from build123d import *

# Parameters (mm, degrees)
SKETCH_1_R          = 14
SKETCH_1_R_2        = 8.2
EXTRUDE_1_DEPTH     = 6
EXTRUDE_2_DEPTH     = 16
SKETCH_3_R          = 1.7
CUT_EXTRUDE_1_DEPTH = 34.540015912
SKETCH_4_R          = 1.5
CUT_EXTRUDE_2_DEPTH = 34.540015912
CUT_EXTRUDE_3_DEPTH = 13
CHAMFER_1_SIZE      = 3
CHAMFER_2_SIZE      = 1


with BuildPart() as part:
    # 草圖1 → 填料-伸長1 (new body)
    with BuildSketch(Plane.XY):
        Circle(SKETCH_1_R)
        Circle(SKETCH_1_R_2, mode=Mode.SUBTRACT)
    extrude(amount=EXTRUDE_1_DEPTH)

    # 草圖2 → 填料-伸長2 (add)
    with BuildSketch(Plane.XY):
        with BuildLine():
            Line((20.686533479, -6.169872981), (13.824751653, -2.208221396))
            ThreePointArc((13.824751653, -2.208221396), (12.124355653, -7), (8.824751653, -10.868475434))
            Line((8.824751653, -10.868475434), (15.686533479, -14.830127019))
            Line((15.686533479, -14.830127019), (20.686533479, -6.169872981))
        make_face()
        with BuildLine():
            Line((-5, 21), (5, 21))
            Line((5, 21), (5, 13.076696831))
            ThreePointArc((5, 13.076696831), (0, 14), (-5, 13.076696831))
            Line((-5, 13.076696831), (-5, 21))
        make_face()
        with BuildLine():
            Line((-15.686533479, -14.830127019), (-8.824751653, -10.868475434))
            ThreePointArc((-8.824751653, -10.868475434), (-12.124355653, -7), (-13.824751653, -2.208221396))
            Line((-13.824751653, -2.208221396), (-20.686533479, -6.169872981))
            Line((-20.686533479, -6.169872981), (-15.686533479, -14.830127019))
        make_face()
    extrude(amount=EXTRUDE_2_DEPTH)

    # 草圖3 → 除料-伸長1 (cut, through all)
    with BuildSketch(Plane.XY.offset(16)):
        with Locations((0, 18)):
            Circle(SKETCH_3_R)
        with Locations((15.588457268, -9)):
            Circle(SKETCH_3_R)
        with Locations((-15.588457268, -9)):
            Circle(SKETCH_3_R)
    extrude(amount=-CUT_EXTRUDE_1_DEPTH, mode=Mode.SUBTRACT)

    # 草圖4 → 除料-伸長2 (cut, through all)
    with BuildSketch(Plane(origin=(0, 0, 0), x_dir=(-1, 0, 0), z_dir=(0, 0, -1))):
        with Locations((0, 11)):
            Circle(SKETCH_4_R)
        with Locations((9.526279442, -5.5)):
            Circle(SKETCH_4_R)
        with Locations((-9.526279442, -5.5)):
            Circle(SKETCH_4_R)
    extrude(amount=-CUT_EXTRUDE_2_DEPTH, mode=Mode.SUBTRACT)

    # 草圖5 → 除料-伸長3 (cut)
    with BuildSketch(Plane(origin=(0, 0, 0), x_dir=(-1, 0, 0), z_dir=(0, 0, -1))):
        with BuildLine():
            Line((17.088457268, -6.401923789), (19.686533479, -7.901923789))
            Line((19.686533479, -7.901923789), (16.686533479, -13.098076211))
            Line((16.686533479, -13.098076211), (14.088457268, -11.598076211))
            ThreePointArc((14.088457268, -11.598076211), (12.990381057, -7.5), (17.088457268, -6.401923789))
        make_face()
        with BuildLine():
            Line((-3, 18), (-3, 21))
            Line((-3, 21), (3, 21))
            Line((3, 21), (3, 18))
            ThreePointArc((3, 18), (0, 15), (-3, 18))
        make_face()
        with BuildLine():
            Line((-14.088457268, -11.598076211), (-16.686533479, -13.098076211))
            Line((-16.686533479, -13.098076211), (-19.686533479, -7.901923789))
            Line((-19.686533479, -7.901923789), (-17.088457268, -6.401923789))
            ThreePointArc((-17.088457268, -6.401923789), (-12.990381057, -7.5), (-14.088457268, -11.598076211))
        make_face()
    extrude(amount=-CUT_EXTRUDE_3_DEPTH, mode=Mode.SUBTRACT)

    # 導角1
    chamfer_1_edges = [part.edges().sort_by_distance(p)[0] for p in [
        (4, 21, 0),
        (-4, 21, 0),
        (-20.186533479, -7.035898385, 0),
        (-16.186533479, -13.964101615, 0),
        (20.186533479, -7.035898385, 0),
        (16.186533479, -13.964101615, 0),
    ]]
    chamfer(chamfer_1_edges, length=CHAMFER_1_SIZE)

    # 導角2
    # the kernel refuses this chamfer: 1 mm, written as the material it adds along each edge
    with BuildSketch(Plane(origin=(0, 0, 6), x_dir=(0.4779177917946843, -0.8784045675462375, 0), z_dir=(-0.8784045675462375, -0.4779177917946843, 0))) as chamfer_2_piece_1_section:
        Polygon((14 - CHAMFER_2_SIZE, 0), (14, CHAMFER_2_SIZE), (14, 0), align=None)
    chamfer_2_piece_1 = revolve(axis=Axis((0, 0, 6), (0, 0, 1)), revolution_arc=62.901004407, mode=Mode.PRIVATE)
    chamfer_2_piece_1 = split(chamfer_2_piece_1, bisect_by=Plane(origin=(14.060598585, -2.344387686, 6.333230846), z_dir=(-0.5000000000000002, -0.8660254037844386, 0)), keep=Keep.TOP, mode=Mode.PRIVATE)
    chamfer_2_piece_1 = split(chamfer_2_piece_1, bisect_by=Plane(origin=(9.060598585, -11.004641724, 6.333230846), z_dir=(0.49999999999999956, 0.8660254037844389, 0)), keep=Keep.TOP, mode=Mode.PRIVATE)
    add(chamfer_2_piece_1)
    with BuildSketch(Plane(origin=(0, 0, 6), x_dir=(-0.9996795661926668, 0.025313335158395317, 0), z_dir=(0.025313335158395317, 0.9996795661926668, 0))) as chamfer_2_piece_2_section:
        Polygon((14 - CHAMFER_2_SIZE, 0), (14, CHAMFER_2_SIZE), (14, 0), align=None)
    chamfer_2_piece_2 = revolve(axis=Axis((0, 0, 6), (0, 0, 1)), revolution_arc=62.901004407, mode=Mode.PRIVATE)
    chamfer_2_piece_2 = split(chamfer_2_piece_2, bisect_by=Plane(origin=(-14.060598585, -2.344387686, 6.333230846), z_dir=(0.5000000000000009, -0.8660254037844383, 0)), keep=Keep.TOP, mode=Mode.PRIVATE)
    chamfer_2_piece_2 = split(chamfer_2_piece_2, bisect_by=Plane(origin=(-9.060598585, -11.004641724, 6.333230846), z_dir=(-0.5000000000000003, 0.8660254037844387, 0)), keep=Keep.TOP, mode=Mode.PRIVATE)
    add(chamfer_2_piece_2)
    with BuildSketch(Plane(origin=(0, 0, 6), x_dir=(0.5217617743979716, 0.853091232387885, 0), z_dir=(0.853091232387885, -0.5217617743979716, 0))) as chamfer_2_piece_3_section:
        Polygon((14, CHAMFER_2_SIZE), (14 - CHAMFER_2_SIZE, 0), (14, 0), align=None)
    chamfer_2_piece_3 = revolve(axis=Axis((0, 0, 6), (0, 0, 1)), revolution_arc=62.901004407, mode=Mode.PRIVATE)
    chamfer_2_piece_3 = split(chamfer_2_piece_3, bisect_by=Plane(origin=(5, 13.34902941, 6.333230846), z_dir=(-1, 0, 0)), keep=Keep.TOP, mode=Mode.PRIVATE)
    chamfer_2_piece_3 = split(chamfer_2_piece_3, bisect_by=Plane(origin=(-5, 13.34902941, 6.333230846), z_dir=(1, 0, 0)), keep=Keep.TOP, mode=Mode.PRIVATE)
    add(chamfer_2_piece_3)


solid = part.part
Part model, mm, in its own coordinate system. A direction names the side the tool comes from. Coordinates: 2 decimals unless noted, no trailing zeros. Order: outer loops, then holes, each group sorted by start corner. A loop starts at its lowest first (then second) coordinate and runs counter-clockwise, first axis right, second up. Notation, with made-up numbers: (-8.75, -32.75) - (30.25, -32.75) arc R20 ccw to (30.25, -20.75) - close; hole circle Ø6 at (4.5, 71). An arc over 180 degrees is marked (long way). Use CSV: the item, a comma, the result in double quotes.
Item 1: Saw through at A-A on x = 0. Give the cut face in (y, z).
Solved:
outline,"(-14, 0) - (-8.2, 0) - (-8.2, 6) - (-14, 6) - close; (8.2, 0) - (9.5, 0) - (9.5, 6) - (8.2, 6) - close; (12.5, 0) - (15, 0) - (15, 13) - (16.3, 13) - (16.3, 16) - (14, 16) - (14, 7) - (13, 6) - (12.5, 6) - close; (19.7, 13) - (21, 13) - (21, 16) - (19.7, 16) - close"
Item 2: Saw through at D-D on y = 11. Give the cut face in (x, z), and give its area (3 significant figures).
Solved:
outline,"(-8.66, 0) - (-1.5, 0) - (-1.5, 6) - (-8.66, 6) - close; (1.5, 0) - (8.66, 0) - (8.66, 6) - (1.5, 6) - close"
area,"85.9 mm²"
Item 3: Drop flat-ended pins along their axis: P1, Ø2.5, axis at x = -9.53, y = -5.5, coming from the +Z side; P2, Ø4, axis at x = 0, y = 18, coming from the -Z side; P3, Ø5, axis at x = -0.5, z = 3, coming from the -Y side; P4, Ø1, axis at x = 12.5, y = 3.5, coming from the +Z side. Give the stop position or say it passes through.
Solved:
P1,"passes through"
P2,"stops at z = 13"
P3,"stops at y = -14"
P4,"stops at z = 6"
Item 4: Saw through at C-C on y = -9. Give the number of separate pieces and of enclosed holes in the cut face, and give its area (3 significant figures).
Solved:
separate pieces,"3"
enclosed holes,"0"
area,"208 mm²"
Item 5: 3-axis set-ups, long thin cutter, end or side, ignore diameter. For faces 4 (the face through (-17, -10.3, 13)), 5 (the face through (15.37, -12.34, 7.85)), 6 (the face through (6, 6, 6)): which of +Z, -Z, +X, -X, +Y, -Y reach the whole face in a straight line?
Solved:
face 4,"-Z"
face 5,"-Z, +X"
face 6,"+Z"
Item 6: Probe probe 1 along Y at (x, z) = (0, 13.85); probe 2 along X at (y, z) = (-7, 9.5); probe 3 along X at (y, z) = (20, 12.5). List the from-to ranges inside material, lowest first.
Solved:
probe 1,"y = 14 to 16.3, 19.7 to 21"
probe 2,"x = -20.21 to -18.12, -13.35 to -12.12, 12.12 to 13.35, 18.12 to 20.21"
probe 3,"x = -5 to -3, 3 to 5"
Item 7: Saw through at B-B on y = 1.5. Give the cut face in (x, z), and give its area (3 significant figures).
Solved:
outline,"(-13.92, 0) - (-8.06, 0) - (-8.06, 6) - (-13.92, 6) - close; (8.06, 0) - (13.92, 0) - (13.92, 6) - (8.06, 6) - close"
area,"70.3 mm²"
Item 8: Mould opens along Y. For faces 1 (the face through (13.89, -8.93, 14.52)), 2 (the face through (12.16, -6.94, 11.44)), 3 (the face through (-14, -8, 16)) say: +Y half, -Y half, draft (parallel to the pull), parting line (faces both ways), or undercut.
Solved:
face 1,"undercut"
face 2,"+Y half"
face 3,"draft"
